Input: part model. Units: mm. Frame: model coordinates. A direction names the side the tool comes from. Coordinates: 2 decimals unless noted, no trailing zeros. Write each loop counter-clockwise with the first axis right and the second up, starting at its lowest first coordinate (ties: lowest second). Pieces come first, ordered by that corner, then holes. Notation, with made-up numbers: M 70.5,49 L 107.5,49 A8 ccw 107.5,56 Z; hole C 64,26.5 d3. An arc over 180 degrees is marked long. Use CSV: the item, a comma, the result in double quotes.
Autodesk Inventor part; units mm, degrees
ref_plane "YZ Plane" through (0, 0, 0) normal (1, 0, 0) x (0, 1, 0)
ref_plane "XZ Plane" through (0, 0, 0) normal (0, 1, 0) x (-1, 0, 0)
ref_plane "XY Plane" through (0, 0, 0) normal (0, 0, 1) x (1, 0, 0)
sketch "Sketch2" plane through (0, 0, 0) normal (0, 0, 1) x (1, 0, 0)
  circle A0 centre (0, 0) radius 22.225
  dimension "d4" = 44.45
extrude "Extrusion2" add sketch "Sketch2" along normal blind 4
sketch "Sketch3" plane through (0, 0, 4) normal (0, 0, 1) x (1, 0, 0)
  circle A0 centre (0, 0) radius 22.225
  circle A1 centre (0, 0) radius 17.4625
  dimension "d7" = 34.925
extrude "Extrusion3" add sketch "Sketch3" along normal blind 4.7625 contours A1
sketch "Sketch4" plane through (0, 0, 8.7625) normal (0, 0, 1) x (1, 0, 0)
  circle A0 centre (0, 0) radius 17.4625
  circle A1 centre (0, 0) radius 22.225
  dimension "d10" = 44.45
extrude "Extrusion4" add sketch "Sketch4" along normal blind 4 contours A0 | A1
sketch "Sketch5" plane through (0, 0, 12.7625) normal (0, 0, 1) x (1, 0, 0)
  circle A0 centre (0, 0) radius 22.225
  circle A1 centre (0, 0) radius 17.4625
  dimension "d13" = 34.925
extrude "Extrusion5" add sketch "Sketch5" along normal blind 4.7625 contours A1
sketch "Sketch6" plane through (0, 0, 17.525) normal (0, 0, 1) x (1, 0, 0)
  circle A0 centre (0, 0) radius 17.4625
  circle A1 centre (0, 0) radius 22.225
  dimension "d16" = 44.45
extrude "Extrusion6" add sketch "Sketch6" along normal blind 12 contours A0 | A1
sketch "Sketch7" plane through (0, 0, 29.525) normal (0, 0, 1) x (1, 0, 0)
  circle A0 centre (0, 0) radius 22.225
  circle A1 centre (0, 0) radius 25.4
  dimension "d19" = 50.8
extrude "Extrusion7" add sketch "Sketch7" along normal blind 4 contours A0 | A1
sketch "Sketch8" plane through (0, 0, 33.525) normal (0, 0, 1) x (1, 0, 0)
  circle A0 centre (0, 0) radius 25.4
  circle A1 centre (0, 0) radius 17.4
  dimension "d22" = 34.8
extrude "Extrusion8" add sketch "Sketch8" along normal blind 12 contours A1
sketch "Sketch Main" plane through (0, 0, 45.525) normal (0, 0, 1) x (1, 0, 0)
  circle A0 centre (0, 0) radius 17.4
  circle A1 centre (0, 0) radius 25.4
  line L0 (-17.4, 0) -> (17.4, 0) construction
  circle A2 centre (-9.7141, 0) radius 2.75
  circle A3 centre (-9.7141, 0) radius 4.5
  circle A4 centre (4.7812, 0) radius 6
  circle A5 centre (4.7812, 0) radius 9 construction
  circle A6 centre (4.7812, 0) radius 10 construction
  line L1 (13.4415, 5) -> (13.4415, -5)
  line L2 (13.4415, -5) -> (4.7812, -10)
  line L3 (4.7812, -10) -> (-3.879, -5)
  line L4 (-3.879, -5) -> (-3.879, 5)
  line L5 (-3.879, 5) -> (4.7812, 10)
  line L6 (4.7812, 10) -> (13.4415, 5)
  circle A7 centre (4.7812, 0) radius 1.5
  dimension "d51" = 20
  dimension "d25" = 50.8
  dimension "d39" = 5.5
  dimension "d40" = 9
  dimension "d41" = 12
  dimension "d42" = 18
  dimension "d56" = 3
extrude "Extrusion9" add sketch "Sketch Main" along normal blind 4 contours A0 | A1 | A2 | A3 | A4 | L1 L2 L3 L4 L5 L6 | A7
extrude "Extrusion13" cut sketch "Sketch Main" along normal blind 4 and the other way blind 16 contours A2 | A3
extrude "Extrusion14" cut sketch "Sketch Main" against normal through all contours A2
extrude "Extrusion15" cut sketch "Sketch Main" against normal blind 12 contours A4 | L1 L2 L3 L4 L5 L6 | A7
extrude "Extrusion16" cut sketch "Sketch Main" along normal through all contours A4 | A7
extrude "Extrusion17" cut sketch "Sketch Main" against normal through all contours A7
sketch "Sketch11" plane through (0, 0, 0) normal (0, 0, -1) x (-1, 0, 0)
  circle A0 centre (9.7141, 0) radius 2.75
  circle A1 centre (9.7141, 0) radius 4.5
  dimension "d59" = 9
extrude "Extrusion18" cut sketch "Sketch11" against normal blind 20 contours A0 | A1
properties part number "battery_cap"
1. Contact query for flat-ended pins moving along their axis: pin 1 Ø3 at (x, z) = (-3, 8) entering from -Y; pin 2 Ø3 at (y, z) = (0, 40.5) entering from +X; pin 3 Ø1 at (y, z) = (-0.5, 5) entering from +X. Output: stop coordinate, or through.
Resolved:
pin 1,"stops at y = -22.16"
pin 2,"stops at x = 17.4"
pin 3,"stops at x = 17.46"
2. Section C-C (y = 0). State how many separate pieces and enclosed holes the cut face has, then the cut area to 3 significant figures.
Resolved:
separate pieces,"3"
enclosed holes,"0"
area,"1,280 mm^2"
3. Mould query, pull axis Z, two halves, no side actions, for faces 1 (the cylindrical face through (3.283, 0.066, 16.997)), 2 (the flat face through (0, -5, 49.525)), 3 (the flat face through (0.512, -7.535, 39.609)), 4 (the flat face through (5, -17, 45.525)). Classes: pulls with the +Z half, pulls with the -Z half, needs draft (parallel to the pull), parting line crosses it, or undercut.
Resolved:
face 1,"needs draft"
face 2,"pulls with the +Z half"
face 3,"undercut"
face 4,"undercut"
4. Material intervals for line 1 (Z direction, x = 1, y = -18) (1 decimal); line 2 (Z direction, x = 14, y = 20) (3 decimals); line 3 (Y direction, x = 1.5, z = 45), sorted ascending. Write a range as [from, to].
Resolved:
line 1,"z = [0, 4], [8.8, 12.8], [17.5, 33.5], [45.5, 49.5]"
line 2,"z = [29.525, 33.525], [45.525, 49.525]"
line 3,"y = [-17.34, -8.11], [8.11, 17.34]"
5. Access query for faces 5 (the cylindrical face through (21.199, -6.676, 10.734)), 6 (the flat face through (0, 0, 0)), 7 (the flat face through (10, -15, 4)). Directions: +Z, -Z, +X, -X, +Y, -Y. A direction counts if a zero-diameter tool reaches every point of the face in a straight line with its end or side. Return the directions, or none.
Resolved:
face 5,"-Z"
face 6,"-Z, +X, -X, +Y, -Y"
face 7,"none"
6. Section B-B (x = 19.5). Return loops of the section in (y, z) (1 decimal), then the cut area to 3 significant figures.
Resolved:
outline,"M -16.3,29.5 L -10.7,29.5 L -10.7,17.5 L 10.7,17.5 L 10.7,29.5 L 16.3,29.5 L 16.3,33.5 L -16.3,33.5 Z; M -16.3,45.5 L 16.3,45.5 L 16.3,49.5 L -16.3,49.5 Z; M -10.7,0 L 10.7,0 L 10.7,4 L -10.7,4 Z; M -10.7,8.8 L 10.7,8.8 L 10.7,12.8 L -10.7,12.8 Z"
area,"687 mm^2"
7. Section A-A (z = 44.5). Return loops of the section in (x, y).
Resolved:
outline,"C 0,0 d34.8; hole C -9.71,0 d9; hole M -3.88,-5 L 4.78,-10 L 13.44,-5 L 13.44,5 L 4.78,10 L -3.88,5 Z"
8. Section D-D (y = -21). Return loops of the section in (x, z) (1 decimal).
Resolved:
outline,"M -14.3,29.5 L -7.3,29.5 L -7.3,17.5 L 7.3,17.5 L 7.3,29.5 L 14.3,29.5 L 14.3,33.5 L -14.3,33.5 Z; M -14.3,45.5 L 14.3,45.5 L 14.3,49.5 L -14.3,49.5 Z; M -7.3,0 L 7.3,0 L 7.3,4 L -7.3,4 Z; M -7.3,8.8 L 7.3,8.8 L 7.3,12.8 L -7.3,12.8 Z"
